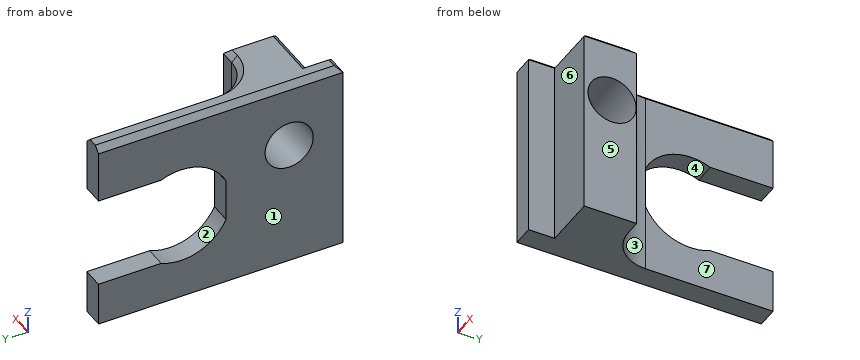
from build123d import *

# Parameters (mm, degrees)
F1_DEPTH = 25.4
F2_R     = 5.08
F3_SIZE  = 0.762
F5_DEPTH = 25.4
F7_D     = 6.35


with BuildPart() as f1:
    # F0 (on Top) → F1 (new body)
    with BuildSketch(Plane.XY):
        Polygon((35.7818603516, 26.3504646719), (35.7818603516, 48.246845603), (32.9955667257, 48.246845603), (32.9955667257, 15.984505415), (35.7818603516, 15.984505415), (35.7818603516, 19.4336399436), (42.8418815136, 19.4336399436), (42.8418815136, 26.3504646719), align=None)
    extrude(amount=F1_DEPTH)

    # F2
    f2_edges = [f1.edges().sort_by_distance(p)[0] for p in [
        (35.78186, 26.350465, 12.7),
    ]]
    fillet(f2_edges, radius=F2_R)

    # F3
    f3_edges = [f1.edges().sort_by_distance(p)[0] for p in [
        (35.78186, 39.838655, 25.4),
        (42.841882, 22.892052, 25.4),
        (39.311871, 19.43364, 25.4),
        (35.78186, 17.709073, 25.4),
        (34.388714, 15.984505, 25.4),
        (32.995567, 32.115676, 25.4),
        (37.269758, 27.838362, 25.4),
        (41.851871, 26.350465, 25.4),
    ]]
    chamfer(f3_edges, length=F3_SIZE)

    # F4 (on face) → F5 (cut)
    with BuildSketch(Plane.YZ.offset(35.7818603516)):
        with BuildLine():
            Line((48.246845603, 5.7491324842), (48.246845603, 17.8127139807))
            Line((48.246845603, 17.8127139807), (39.9765420257, 17.8127139807))
            ThreePointArc((39.9765420257, 17.8127139807), (35.0432489169, 17.9167289348), (31.4304646719, 14.5557781754))
            Line((31.4304646719, 14.5557781754), (31.4304646719, 9.0060682895))
            ThreePointArc((31.4304646719, 9.0060682895), (35.0432489169, 5.6451175301), (39.9765420257, 5.7491324842))
            Line((39.9765420257, 5.7491324842), (48.246845603, 5.7491324842))
        make_face()
    extrude(amount=-F5_DEPTH, mode=Mode.SUBTRACT)

    # F7 (through all)
    with Locations(Plane.YZ.offset(42.8418815136)):
        with Locations((23.1040623039, 16.7023018003)):
            Hole(F7_D / 2)


solid = f1.part
Could you check a few things on this model? Use its own coordinates, in mm. Face numbers are marked on the shaded views. A direction names the side the tool comes from. Round coordinates to 2 decimals unless told otherwise and drop trailing zeros. Loops run counter-clockwise (first coordinate to the right, second up) from the corner with the lowest first, then second, coordinate; pieces in that order, holes last. Notation, with made-up numbers: (1, 51) - (55, 51) arc R36 cw to (55, 87) - close; hole circle Ø6 at (53, 58.25). An arc over 180 degrees is marked (long way). Write item = value, one per line.
1) On a 3-axis mill with a long thin cutter (end or side, diameter ignored), from which of +Z, -Z, +X, -X, +Y, -Y can I reach the whole of each face in a straight line? I mean the marked faces 5, 6 and 7. Say none if no direction works.
Computed:
face_5 = +Z, -Z, +X, +Y, -Y
face_6 = +Z, -Z, +X, -Y
face_7 = +Z, -Z, +X, +Y
2) If we mould it in two halves opening along Y, with no side actions, what happens to the marked faces 1, 2, 3 and 4? For each: pulls with the +Y half, pulls with the -Y half, needs draft (parallel to the pull), parting line crosses it, or undercut.
Computed:
face_1 = needs draft
face_2 = undercut
face_3 = pulls with the +Y half
face_4 = undercut
3) I'm going to push flat-ended pins straight in: P1, Ø5, axis at y = 37, z = 21.5, coming from the +X side; P2, Ø1, axis at x = 38, z = 21, coming from the +Y side; P3, Ø0.8, axis at x = 34, z = 10.5, coming from the +Y side. Where does each tip first touch, or does it pass through?
Computed:
P1 = 35.78
P2 = 27.62
P3 = 31.43
4) Imagine slicing it at B-B (z = 13). Please give me the cut outline in (x, y).
Computed:
outline = (33, 15.98) - (35.78, 15.98) - (35.78, 19.43) - (42.84, 19.43) - (42.84, 26.35) - (40.86, 26.35) arc R5.08 cw to (35.78, 31.43) - (33, 31.43) - close
5) Imagine slicing it at A-A (y = 38). Please give me the cut outline in (x, z), and give its area (3 significant figures).
Computed:
outline = (33, 0) - (35.78, 0) - (35.78, 5.24) - (33, 5.24) - close; (33, 18.32) - (35.78, 18.32) - (35.78, 24.64) - (35.02, 25.4) - (33.76, 25.4) - (33, 24.64) - close
area = 33.8 mm2
6) Imagine slicing it at C-C (y = 42.5). Please give me the cut outline in (x, z).
Computed:
outline = (33, 0) - (35.78, 0) - (35.78, 5.75) - (33, 5.75) - close; (33, 17.81) - (35.78, 17.81) - (35.78, 24.64) - (35.02, 25.4) - (33.76, 25.4) - (33, 24.64) - close
7) I need wall thicknesses on line 1 along X through (y, z) = (35, 5.5); line 2 along Z through (x, y) = (41, 22.5); line 3 along Z through (x, y) = (41.5, 23.5). Which ranges of each line are inside material? Lowest first, please. Write a range as from..to.
Computed:
line_1 = 33..35.78
line_2 = 0..13.59, 19.82..25.4
line_3 = 0..13.55, 19.85..25.4
8) Imagine slicing it at D-D (z = 6.25). Please give me the cut outline in (x, y), and give its area (3 significant figures).
Computed:
outline = (33, 15.98) - (35.78, 15.98) - (35.78, 19.43) - (42.84, 19.43) - (42.84, 26.35) - (40.86, 26.35) arc R5.08 cw to (35.78, 31.43) - (35.78, 33.84) - (33, 33.84) - close
area = 104 mm2
